The drawing under review shows one solid part. Ordinate dimensions are in mm from its lowest x, y, z. Round coordinates to 2 decimals unless told otherwise and drop trailing zeros. Order: outer loops, then holes, each group sorted by start corner. A loop starts at its lowest first (then second) coordinate and runs counter-clockwise, first axis right, second up. Notation, with made-up numbers: (17, 78) - (52, 78) arc R14 cw to (52, 85) - close; hole circle Ø3 at (-12, 20). An arc over 180 degrees is marked (long way). Answer as a JSON object with one key per item and string values. Group by question number.
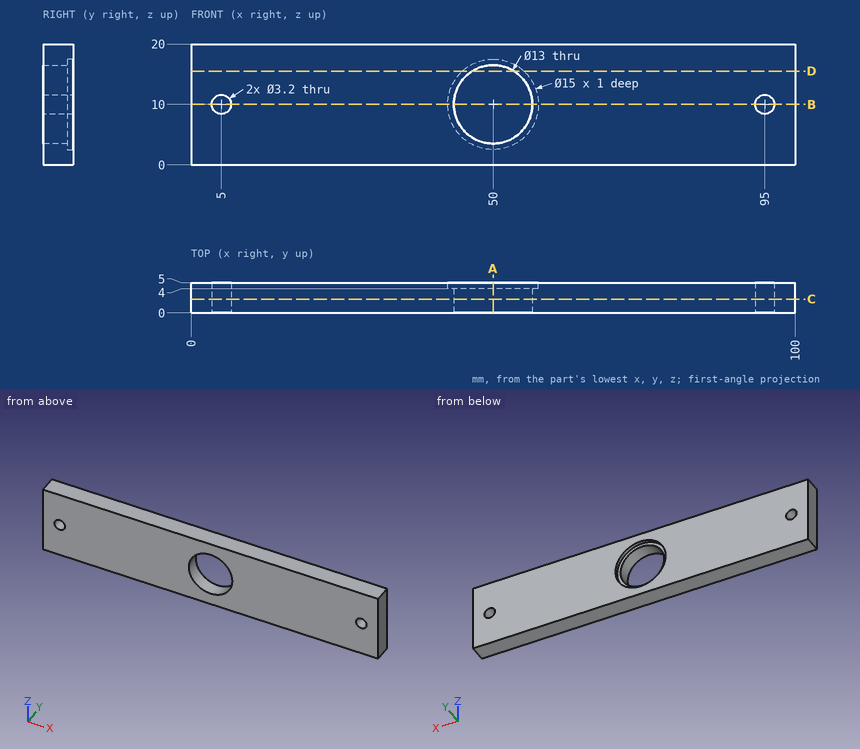
1. Take a section at B-B, the plane z = 10. Give the boundary of the cut face in (x, y).
2. Take a section at D-D, the plane z = 15.5. Give the boundary of the cut face in (x, y), then the cut area to 3 significant figures.
3. Take a section at A-A, the plane x = 50. Give the boundary of the cut face in (y, z).
4. To check wall thickness, follow line 1 (X direction, y = 2.3, z = 10); line 2 (X direction, y = 4.55, z = 10); line 3 (Z direction, x = 50, y = 2.55). State the ranges of each line that lie inside material, in increasing order. Write a range as from..to.
5. Clearance check with a flat-ended pin moving along its axis: P1, Ø4, axis at x = 29, z = 7, coming from the -Y side. State where the tip first meets the part, or that it passes through.
6. Take a section at C-C, the plane y = 2.3. Give the boundary of the cut face in (x, z), then the cut area to 3 significant figures.
Response values:
{
 "1": {"outline": "(0, 0) - (3.4, 0) - (3.4, 5) - (0, 5) - close; (6.6, 0) - (43.5, 0) - (43.5, 4) - (42.5, 4) - (42.5, 5) - (6.6, 5) - close; (56.5, 0) - (93.4, 0) - (93.4, 5) - (57.5, 5) - (57.5, 4) - (56.5, 4) - close; (96.6, 0) - (100, 0) - (100, 5) - (96.6, 5) - close"},
 "2": {"outline": "(0, 0) - (46.54, 0) - (46.54, 4) - (44.9, 4) - (44.9, 5) - (0, 5) - close; (53.46, 0) - (100, 0) - (100, 5) - (55.1, 5) - (55.1, 4) - (53.46, 4) - close", "area": "462 mm2"},
 "3": {"outline": "(0, 0) - (5, 0) - (5, 2.5) - (4, 2.5) - (4, 3.5) - (0, 3.5) - close; (0, 16.5) - (4, 16.5) - (4, 17.5) - (5, 17.5) - (5, 20) - (0, 20) - close"},
 "4": {"line 1": "0..3.4, 6.6..43.5, 56.5..93.4, 96.6..100", "line 2": "0..3.4, 6.6..42.5, 57.5..93.4, 96.6..100", "line 3": "0..3.5, 16.5..20"},
 "5": {"P1": "y = 0"},
 "6": {"outline": "(0, 0) - (100, 0) - (100, 20) - (0, 20) - close; hole circle Ø3.2 at (5, 10); hole circle Ø13 at (50, 10); hole circle Ø3.2 at (95, 10)", "area": "1,850 mm2"}
}
